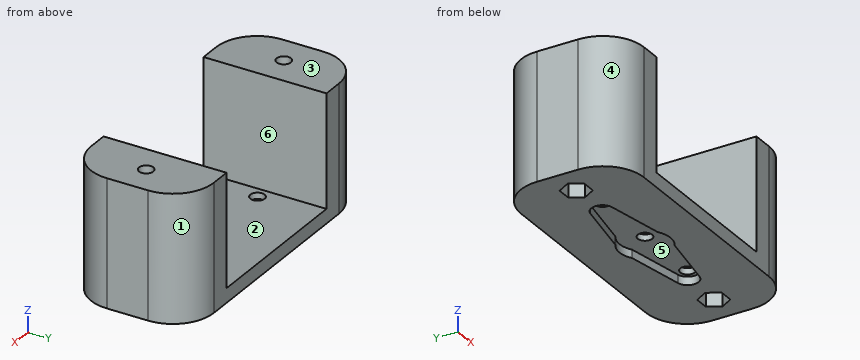
from build123d import *

# Parameters (mm, degrees)
BOSS_EXTRUDE1_DEPTH = 31
SKETCH2_W           = 40
SKETCH2_H           = 30
CUT_EXTRUDE1_DEPTH  = 27.5
SKETCH3_R           = 1.75
CUT_EXTRUDE2_DEPTH  = 32
CUT_EXTRUDE3_DEPTH  = 5
CUT_EXTRUDE4_DEPTH  = 2
SKETCH6_R           = 1.75
CUT_EXTRUDE5_DEPTH  = 32


with BuildPart() as part:
    # Sketch1 → Boss-Extrude1 (new body)
    with BuildSketch(Plane.XY):
        with BuildLine():
            Line((-25, 15), (25, 15))
            ThreePointArc((25, 15), (32.071067812, 12.071067812), (35, 5))
            Line((35, 5), (35, -5))
            ThreePointArc((35, -5), (32.071067812, -12.071067812), (25, -15))
            Line((25, -15), (-25, -15))
            ThreePointArc((-25, -15), (-32.071067812, -12.071067812), (-35, -5))
            Line((-35, -5), (-35, 5))
            ThreePointArc((-35, 5), (-32.071067812, 12.071067812), (-25, 15))
        make_face()
    extrude(amount=BOSS_EXTRUDE1_DEPTH)

    # Sketch2 → Cut-Extrude1 (cut)
    with BuildSketch(Plane.XY.offset(31)):
        Rectangle(SKETCH2_W, SKETCH2_H)
    extrude(amount=-CUT_EXTRUDE1_DEPTH, mode=Mode.SUBTRACT)

    # Sketch3 → Cut-Extrude2 (cut, through all)
    with BuildSketch(Plane.XY.offset(31)):
        with Locations((-27.5, 0)):
            Circle(SKETCH3_R)
        with Locations((27.5, 0)):
            Circle(SKETCH3_R)
    extrude(amount=-CUT_EXTRUDE2_DEPTH, mode=Mode.SUBTRACT)

    # Sketch4 → Cut-Extrude3 (cut)
    with BuildSketch(Plane(origin=(0, 0, 0), x_dir=(-1, 0, 0), z_dir=(0, 0, -1))):
        Polygon((-24.035898385, 0), (-25.767949192, 3), (-29.232050808, 3), (-30.964101615, 0), (-29.232050808, -3), (-25.767949192, -3), align=None)
        Polygon((24.035898385, 0), (25.767949192, -3), (29.232050808, -3), (30.964101615, 0), (29.232050808, 3), (25.767949192, 3), align=None)
    extrude(amount=-CUT_EXTRUDE3_DEPTH, mode=Mode.SUBTRACT)

    # Sketch5 → Cut-Extrude4 (cut)
    with BuildSketch(Plane(origin=(0, 0, 0), x_dir=(-1, 0, 0), z_dir=(0, 0, -1))):
        with BuildLine():
            Line((-17.477732777, -2.657399367), (-3.39236806, -5.189589478))
            ThreePointArc((-3.39236806, -5.189589478), (0, -6.2), (3.39236806, -5.189589478))
            Line((3.39236806, -5.189589478), (17.477732777, -2.657399367))
            ThreePointArc((17.477732777, -2.657399367), (19.7, 0), (17.477732777, 2.657399367))
            Line((17.477732777, 2.657399367), (3.39236806, 5.189589478))
            ThreePointArc((3.39236806, 5.189589478), (0, 6.2), (-3.39236806, 5.189589478))
            Line((-3.39236806, 5.189589478), (-17.477732777, 2.657399367))
            ThreePointArc((-17.477732777, 2.657399367), (-19.7, 0), (-17.477732777, -2.657399367))
        make_face()
    extrude(amount=-CUT_EXTRUDE4_DEPTH, mode=Mode.SUBTRACT)

    # Sketch6 → Cut-Extrude5 (cut, through all)
    with BuildSketch(Plane(origin=(0, 0, 0), x_dir=(-1, 0, 0), z_dir=(0, 0, -1))):
        Circle(SKETCH6_R)
        with Locations((-17, 0)):
            Circle(SKETCH6_R)
        with Locations((17, 0)):
            Circle(SKETCH6_R)
    extrude(amount=-CUT_EXTRUDE5_DEPTH, mode=Mode.SUBTRACT)


solid = part.part
Build history of the part. All positions in model axes, mm. Face numbers are marked on the shaded views. A direction names the side the tool comes from. Coordinates: 2 decimals unless noted, no trailing zeros. Write each loop counter-clockwise with the first axis right and the second up, starting at its lowest first coordinate (ties: lowest second). Pieces come first, ordered by that corner, then holes.
(1) Cut at B-B on x = -27.5. List the corners of the cut face in (y, z), and give its area (3 significant figures).
(2) Mould opens along X. For the marked faces 1, 2 and 3 say: pulls with the +X half, pulls with the -X half, needs draft (parallel to the pull), parting line crosses it, or undercut.
(3) Cut at A-A on z = 19.5. List the corners of the cut face in (x, y), and give its area (3 significant figures).
(4) 3-axis set-ups, long thin cutter, end or side, ignore diameter. For the marked faces 4, 5 and 6: which of +Z, -Z, +X, -X, +Y, -Y reach the whole face in a straight line?
(5) Cut at D-D on x = -10.5. List the corners of the cut face in (y, z), and give its area (3 significant figures).
(6) Drill centre lines: line 1 (X direction, y = 1, z = 10); line 2 (Y direction, x = 0, z = 2.4); line 3 (X direction, y = -5, z = 23.5). Where is each one in solid material? Low to high.
(7) Cut at C-C on y = -7. List the corners of the cut face in (x, z).
(8) Pin check, flat tips, straight feed: pin 1 Ø3 at (x, z) = (28.5, 2.5) entering from +Y; pin 2 Ø4 at (x, y) = (4.5, 1.5) entering from +Z; pin 3 Ø3 at (x, y) = (0, 0) entering from -Z; pin 4 Ø2 at (y, z) = (-8, 26) entering from -X. Stop position of each tip, or through.
Working result:
1. outline: (-14.68, 0) - (-3, 0) - (-3, 5) - (-1.75, 5) - (-1.75, 31) - (-14.68, 31) - close; (1.75, 5) - (3, 5) - (3, 0) - (14.68, 0) - (14.68, 31) - (1.75, 31) - close
1. area: 789 mm2
2. face 1: pulls with the +X half
2. face 2: undercut
2. face 3: needs draft
3. outline: (-35, -5) arc R10 ccw to (-25, -15) - (-20, -15) - (-20, 15) - (-25, 15) arc R10 ccw to (-35, 5) - close; (20, -15) - (25, -15) arc R10 ccw to (35, -5) - (35, 5) arc R10 ccw to (25, 15) - (20, 15) - close; hole circle Ø3.5 at (-27.5, 0); hole circle Ø3.5 at (27.5, 0)
3. area: 795 mm2
4. face 4: +Z, -Z, -X, -Y
4. face 5: -Z
4. face 6: +Z, +Y, -Y
5. outline: (-15, 0) - (-3.91, 0) - (-3.91, 2) - (3.91, 2) - (3.91, 0) - (15, 0) - (15, 3.5) - (-15, 3.5) - close
5. area: 89.4 mm2
6. line 1: x = -35 to -28.94, -26.06 to -20, 20 to 26.06, 28.94 to 35
6. line 2: y = -15 to -1.75, 1.75 to 15
6. line 3: x = -35 to -20, 20 to 35
7. outline: (-34.8, 0) - (34.8, 0) - (34.8, 31) - (20, 31) - (20, 3.5) - (-20, 3.5) - (-20, 31) - (-34.8, 31) - close
8. pin 1: stops at y = 14.8
8. pin 2: stops at z = 3.5
8. pin 3: passes through
8. pin 4: stops at x = -34.8
